Design review of the part built by this model. Coordinates are the model's own, in mm. Give positions to 0.01 mm unless a question says otherwise; leave off trailing zeros. Loops run counter-clockwise (first coordinate to the right, second up) from the corner with the lowest first, then second, coordinate; pieces in that order, holes last. Notation, with made-up numbers: M -25.75,71.5 L 29.25,71.5 A17 cw 29.25,80.5 Z; hole C -3,85 d9. An arc over 180 degrees is marked long. Use one line per item in the form item = value. Start each with the question number.
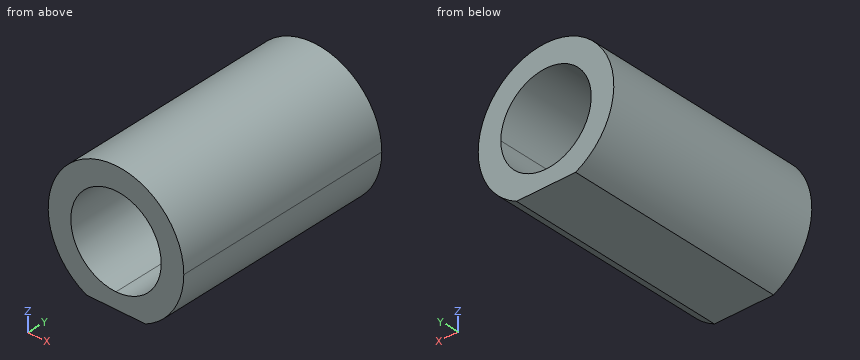
from build123d import *

# Parameters (mm, degrees)
F1_DEPTH = 25
F2_W     = 7.634899
F2_H     = 3.302
F2_W_2   = 7.225763
F3_DEPTH = 181.102


with BuildPart() as f1:
    # F0 (on Front) → F1 (new body)
    with BuildSketch(Plane.XZ):
        with BuildLine():
            ThreePointArc((7.62, 0), (-5.388154, 5.388154), (0, -7.62))
            ThreePointArc((0, -7.62), (5.388154, -5.388154), (7.62, 0))
        make_face()
        with BuildLine():
            ThreePointArc((0, -5.08), (-3.592102, 3.592102), (5.08, 0))
            ThreePointArc((5.08, 0), (3.592102, -3.592102), (0, -5.08))
        make_face(mode=Mode.SUBTRACT)
    extrude(amount=F1_DEPTH)

    # F2 (on Front) → F3 (cut)
    with BuildSketch(Plane.XZ):
        with Locations((3.817449, -8.509)):
            Rectangle(F2_W, F2_H)
        with Locations((-3.612881, -8.509)):
            Rectangle(F2_W_2, F2_H)
    extrude(amount=F3_DEPTH, mode=Mode.SUBTRACT)


solid = f1.part
Q1. Wall thickness on probe 1 along Z at (x, y) = (3.5, -14.5); probe 2 along X at (y, z) = (-14.25, -1.75); probe 3 along X at (y, z) = (-22.5, -0.5): over which ranges is each line inside the solid? List them lowest first.
Q2. Take a section at B-B on x = 1.5. Give the boundary of the cut face in (y, z).
Q3. Take a section at C-C on y = -10. Give the boundary of the cut face in (x, z).
Q4. Clearance check with flat-ended pins moving along their axes: pin 1 Ø1 at (y, z) = (-13.5, 2.5) entering from -X; pin 2 Ø2 at (x, y) = (5, -12) entering from -Z; pin 3 Ø8 at (x, z) = (0, 0) entering from +Y. State where each tip first meets the part, or that it passes through.
Q5. Take a section at D-D on x = -6. Give the boundary of the cut face in (y, z), plus the area to 3 significant figures.
Q6. Take a section at A-A on z = -2.25. Give the boundary of the cut face in (x, y).
Response values:
q1.probe_1 = -6.77 to -3.68, 3.68 to 6.77
q1.probe_2 = -7.42 to -4.77, 4.77 to 7.42
q1.probe_3 = -7.6 to -5.06, 5.06 to 7.6
q2.outline = M -25,-6.86 L 0,-6.86 L 0,-4.85 L -25,-4.85 Z; M -25,4.85 L 0,4.85 L 0,7.47 L -25,7.47 Z
q3.outline = M -3.32,-6.86 L 3.32,-6.86 A7.62 ccw 7.62,0 A7.62 ccw long Z; hole M 0,-5.08 A5.08 ccw 5.08,0 A5.08 ccw long Z
q4.pin_1 = -7.35
q4.pin_2 = -6.49
q4.pin_3 = through
q5.outline = M -25,-4.7 L 0,-4.7 L 0,4.7 L -25,4.7 Z
q5.area = 235 mm^2
q6.outline = M -7.28,-25 L -4.55,-25 L -4.55,0 L -7.28,0 Z; M 4.55,-25 L 7.28,-25 L 7.28,0 L 4.55,0 Z
